Solid Edge part; units mm, degrees
sketch "Sketch1" plane through (0, 0, 0) normal (0, 0, 1) x (1, 0, 0)
  circle A0 centre (0, 0) radius 30
  circle A1 centre (0, 0) radius 2.6
extrude "Protrusion1" add sketch "Sketch1" along normal blind 5
sketch "Sketch2" plane through (0, 0, 5) normal (0, 0, 1) x (1, 0, 0)
  circle A0 centre (-25, 0) radius 4.125
extrude "ExtrudedCutout_1" cut sketch "Sketch2" against normal blind 3
sketch "Sketch3" plane through (0, 0, 5) normal (0, 0, 1) x (1, 0, 0)
  circle A0 centre (-25, 0) radius 5
  circle A1 centre (-25, 0) radius 4.125
extrude "ExtrudedProtrusion_2" add sketch "Sketch3" along normal blind 1.5
sketch "Sketch4" plane through (0, 0, 5) normal (0, 0, 1) x (1, 0, 0)
  circle A0 centre (0, 0) radius 2.6
  circle A1 centre (0, 0) radius 13
extrude "ExtrudedProtrusion_3" add sketch "Sketch4" along normal blind 9
pattern_circular "Pattern1" count 4 over 360 about axis through (0, 0, 0) along (0, 0, -1) of "ExtrudedCutout_1", "ExtrudedProtrusion_2"
sketch "Sketch5" plane through (0, 0, 14) normal (0, 0, 1) x (1, 0, 0)
  circle A0 centre (-8, 0) radius 1.625
  circle A1 centre (0, 8) radius 1.625
  circle A2 centre (8, 0) radius 1.625
  circle A3 centre (0, -8) radius 1.625
extrude "Cutout1" cut sketch "Sketch5" against normal up to next
sketch "Sketch6" plane through (0, 0, 0) normal (0, 0, -1) x (1, 0, 0)
  circle A0 centre (8, 0) radius 2.25
  circle A1 centre (8, 0) radius 1.625
  circle A2 centre (0, -8) radius 2.25
  circle A3 centre (0, -8) radius 1.625
  circle A4 centre (0, 8) radius 2.25
  circle A5 centre (0, 8) radius 1.625
  circle A6 centre (-8, 0) radius 2.25
  circle A7 centre (-8, 0) radius 1.625
extrude "Cutout2" cut sketch "Sketch6" against normal blind 5.25
chamfer "Chamfer_3" distance 0.8 distance2 0.4 4 edges at (-2.25, -8, 5.25) (5.75, 0, 5.25) (-2.25, 8, 5.25) (-10.25, 0, 5.25) measured on face at (1.545, -9.455, 5.25) measured on face at (-6.455, -1.455, 5.25) measured on face at (9.545, -1.455, 5.25) measured on face at (1.545, 6.545, 5.25) measured on face at (1.545, -9.455, 5.25) measured on face at (-6.455, -1.455, 5.25) measured on face at (9.545, -1.455, 5.25) measured on face at (1.545, 6.545, 5.25) measured on face at (1.545, -9.455, 5.25) measured on face at (-6.455, -1.455, 5.25) measured on face at (9.545, -1.455, 5.25) measured on face at (1.545, 6.545, 5.25) measured on face at (1.545, -9.455, 5.25) measured on face at (-6.455, -1.455, 5.25) measured on face at (9.545, -1.455, 5.25) measured on face at (1.545, 6.545, 5.25)
Input: part model. Units: mm. Frame: model coordinates. A direction names the side the tool comes from. Round coordinates to 2 decimals unless told otherwise and drop trailing zeros. Write each loop counter-clockwise with the first axis right and the second up, starting at its lowest first coordinate (ties: lowest second). Pieces come first, ordered by that corner, then holes. Notation, with made-up numbers: (65.5, 24) -> (115.5, 24) arc R19 cw to (115.5, 54) -> close; hole circle Ø5 at (25, 88.5). An arc over 180 degrees is marked (long way). Answer as CSV lines item,"result".
1. Reachability of faces 4 (the cylindrical face through (-1, 21, 4)), 5 (the flat face through (6, -6, 0)), 6 (the cylindrical face through (-10.248, -0.099, 2.391)) from +Z, -Z, +X, -X, +Y, -Y: full face, straight path, thin tool, end or side. Return the list, or none.
Geometry says:
face 4,"+Z"
face 5,"-Z, +X, -X, +Y, -Y"
face 6,"-Z"
2. Section A-A (z = 8). Return the cut outline in (x, y) (3 decimals), plus the area to 3 significant figures.
Geometry says:
outline,"circle Ø26 at (0, 0); hole circle Ø3.25 at (-8, 0); hole circle Ø5.2 at (0, 0); hole circle Ø3.25 at (0, -8); hole circle Ø3.25 at (0, 8); hole circle Ø3.25 at (8, 0)"
area,"477 mm^2"
3. Contact query for flat-ended pins moving along their axis: P1, Ø1.5, axis at y = -13.5, z = 3, coming from the -X side; P2, Ø8, axis at y = -14.5, z = 7.5, coming from the +X side; P3, Ø8, axis at x = -23.5, z = 10, coming from the -Y side; P4, Ø1.9, axis at x = -8, y = 0, coming from the +Z side. Output: stop coordinate, or through.
Geometry says:
P1,"stops at x = -27.16"
P2,"stops at x = 27.76"
P3,"stops at y = -5"
P4,"passes through"
4. Mould query, pull axis Y, two halves, no side actions, for faces 1 (the flat face through (4, 27, 6.5)), 2 (the cylindrical face through (-30, 0, 6)), 3 (the cylindrical face through (-0.29, -10.23, 2.39)). Classes: +Y half, -Y half, draft (parallel to the pull), parting line (faces both ways), or undercut.
Geometry says:
face 1,"draft"
face 2,"parting line"
face 3,"undercut"
5. Section C-C (y = 25). Return the cut outline in (x, z) (3 decimals).
Geometry says:
outline,"(-16.583, 0) -> (16.583, 0) -> (16.583, 5) -> (5, 5) -> (5, 6.5) -> (4.125, 6.5) -> (4.125, 2) -> (-4.125, 2) -> (-4.125, 6.5) -> (-5, 6.5) -> (-5, 5) -> (-16.583, 5) -> close"
6. Ray query, L1, parallel to Y at x = 0, z = 7.5 (3 decimals); L2, parallel to Y at x = 8, z = 11 (3 decimals); L3, parallel to Z at x = -23.5, y = -0.5. Return the intervals inside material, ascending. Write a range as [from, to].
Geometry says:
L1,"y = [-13, -9.625], [-6.375, -2.6], [2.6, 6.375], [9.625, 13]"
L2,"y = [-10.247, -1.625], [1.625, 10.247]"
L3,"z = [0, 2]"
